Read the model definition and answer for the solid it produces. Units are mm, in the model's axes. Face numbers are marked on the shaded views. A direction names the side the tool comes from. Give positions to 0.01 mm unless a question says otherwise; leave off trailing zeros. Write each loop counter-clockwise with the first axis right and the second up, starting at its lowest first coordinate (ties: lowest second). Pieces come first, ordered by that corner, then holes. Notation, with made-up numbers: M -16,82.5 L -12,82.5 A18 cw -12,116.5 Z; hole C 59.25,-29 d10. An arc over 180 degrees is marked long. Put each result on its own line as item: value.
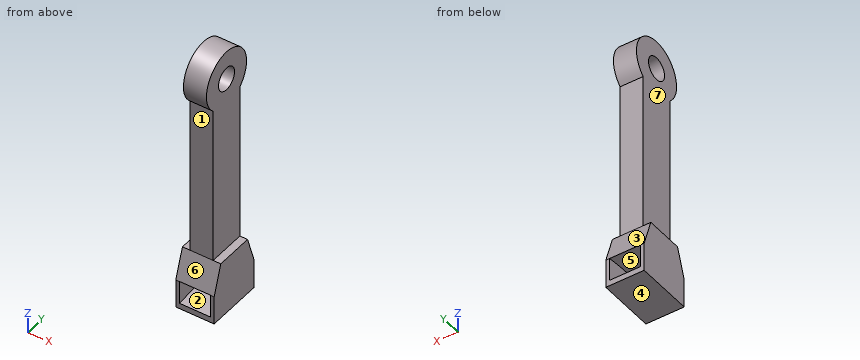
from build123d import *

# Parameters (mm, degrees)
SKETCH1_W               = 10
SKETCH1_H               = 15
BOSS_EXTRUDE1_DEPTH     = 15
CUT_EXTRUDE1_DEPTH      = 30
CUT_EXTRUDE3_DEPTH      = 4
CUT_EXTRUDE3_DEPTH_BACK = 4
CUT_EXTRUDE3_START      = -5
SKETCH13_W              = 10
SKETCH13_H              = 10
BOSS_EXTRUDE2_DEPTH     = 52
SKETCH14_R              = 7.5
SKETCH14_R_2            = 5
BOSS_EXTRUDE3_DEPTH     = 10
SKETCH16_R              = 3
CUT_EXTRUDE4_DEPTH      = 10
CUT_EXTRUDE5_DEPTH      = 10
CUT_EXTRUDE5_DEPTH_BACK = 20
SKETCH17_W              = 2
SKETCH17_H              = 56.751381774
SKETCH17_H_2            = 60.928957135


with BuildPart() as part:
    # Sketch1 → Boss-Extrude1 (new body)
    with BuildSketch(Plane.XY):
        with Locations((5, -7.5)):
            Rectangle(SKETCH1_W, SKETCH1_H)
    extrude(amount=BOSS_EXTRUDE1_DEPTH)

    # Sketch2 → Cut-Extrude1 (cut)
    with BuildSketch(Plane(origin=(10, 0, 0), x_dir=(0, 0, -1), z_dir=(1, 0, 0))):
        Polygon((-7.5, 0), (-15, -2.5), (-15, 0), align=None)
        Polygon((-7.5, -15), (-15, -12.5), (-15, -15), align=None)
    extrude(amount=-CUT_EXTRUDE1_DEPTH, mode=Mode.SUBTRACT)

    # Sketch12 → Cut-Extrude3 (cut, two sides: drawn at the far end of the back side and taken through both)
    with BuildSketch(Plane(origin=(10, 0, 0), x_dir=(0, 0, -1), z_dir=(1, 0, 0)).offset(CUT_EXTRUDE3_START - CUT_EXTRUDE3_DEPTH_BACK)):
        with BuildLine():
            ThreePointArc((7.921073494, 33.458565328), (-8, -7.5), (7.921073494, -48.458565328))
            ThreePointArc((7.921073494, -48.458565328), (12.159622245, -48.644856749), (12.345913666, -44.406307999))
            ThreePointArc((12.345913666, -44.406307999), (-2, -7.5), (12.345913666, 29.406307999))
            ThreePointArc((12.345913666, 29.406307999), (12.159622245, 33.644856749), (7.921073494, 33.458565328))
        make_face()
    extrude(amount=CUT_EXTRUDE3_DEPTH + CUT_EXTRUDE3_DEPTH_BACK, mode=Mode.SUBTRACT)

    # Sketch13 → Boss-Extrude2 (add)
    with BuildSketch(Plane.XY.offset(15)):
        with Locations((5, -7.5)):
            Rectangle(SKETCH13_W, SKETCH13_H)
    extrude(amount=BOSS_EXTRUDE2_DEPTH)

    # Sketch14 → Boss-Extrude3 (add)
    with BuildSketch(Plane.ZY):
        with Locations((62, -7.5)):
            Circle(SKETCH14_R)
        with Locations((62, -7.5)):
            Circle(SKETCH14_R_2, mode=Mode.SUBTRACT)
    extrude(amount=-BOSS_EXTRUDE3_DEPTH)

    # Sketch16 → Cut-Extrude4 (cut)
    with BuildSketch(Plane.ZY):
        with Locations(Location((62, -7.5, 0), (0, 0, 270))):
            Circle(SKETCH16_R)
    extrude(amount=-CUT_EXTRUDE4_DEPTH, mode=Mode.SUBTRACT)

    # Sketch17 → Cut-Extrude5 (cut, two sides: drawn at the far end of the back side and taken through both)
    with BuildSketch(Plane(origin=(0, -2.5, 0), x_dir=(1, 0, 0), z_dir=(0, 1, 0)).offset(-CUT_EXTRUDE5_DEPTH_BACK)):
        with Locations((1, -43.375690887)):
            Rectangle(SKETCH17_W, SKETCH17_H)
        with Locations((9, -45.464478568)):
            Rectangle(SKETCH17_W, SKETCH17_H_2)
    extrude(amount=CUT_EXTRUDE5_DEPTH + CUT_EXTRUDE5_DEPTH_BACK, mode=Mode.SUBTRACT)


solid = part.part
(1) Section D-D on z = 52 is taken. Determine the outline of the cut face in (x, y), and give its area (3 significant figures).
Result:
outline: M 2,-12.5 L 8,-12.5 L 8,-2.5 L 2,-2.5 Z
area: 60.0 mm²
(2) Straight lines are drawn through the part: line 1 along Z through (x, y) = (5.55, -7.5); line 2 along Z through (x, y) = (4.75, -5); line 3 along Y through (x, z) = (7.5, 50). For each, find the intervals that lie inside material, in ascending order. Write a range as from..to.
Result:
line 1: z = 0..2, 8..59, 65..69.5
line 2: z = 0..1.94, 7.95..60.34, 63.66..69.07
line 3: y = -12.5..-2.5
(3) For a pull along Z with two mould halves and no side action, classify the marked faces 4, 5, 6 and 7 as +Z half, -Z half, draft (parallel to the pull), parting line (faces both ways), or undercut.
Result:
face 4: -Z half
face 5: undercut
face 6: undercut
face 7: draft
(4) Which of the six approach directions +Z, -Z, +X, -X, +Y, -Y give full straight-line access (tool end or side, diameter ignored) to the marked faces 1, 2 and 3?
Result:
face 1: +X, -X, -Y
face 2: none
face 3: +X, -X, +Y
(5) Section B-B on y = -7.5 is taken. Determine the outline of the cut face in (x, z), and give its area (3 significant figures).
Result:
outline: M 0,0 L 10,0 L 10,15 L 8,15 L 8,59 L 2,59 L 2,15 L 0,15 Z; M 2,65 L 8,65 L 8,69.5 L 2,69.5 Z; hole M 1,2 L 9,2 L 9,8 L 1,8 Z
area: 393 mm²
(6) Section C-C on z = 62 is taken. Determine the outline of the cut face in (x, y).
Result:
outline: M 2,-15 L 8,-15 L 8,-10.5 L 2,-10.5 Z; M 2,-4.5 L 8,-4.5 L 8,0 L 2,0 Z
(7) Given pin 1 Ø4.5 at (y, z) = (-4.5, 44) entering from +X; pin 2 Ø7.5 at (y, z) = (-6.5, 47) entering from -X; pin 3 Ø1 at (x, y) = (9, -6) entering from +Z, each flat-ended and moving along its own axis, determine where each tip first touches the part or whether it passes through.
Result:
pin 1: stops at x = 8
pin 2: stops at x = 2
pin 3: stops at z = 15
(8) Section A-A on x = 5.75 is taken. Determine the outline of the cut face in (y, z).
Result:
outline: M -15,0 L 0,0 L 0,1.48 A54.65 ccw -15,1.48 Z; M -14.99,7.54 A60.65 cw -0.01,7.54 L -2.5,15 L -2.5,56.41 A7.5 ccw long -12.5,56.41 L -12.5,15 Z; hole C -7.5,62 d6
